Geometry: see drawing. Coordinates: mm, zero at the bounding-box minimum. A direction names the side the tool comes from. Coordinates: 2 decimals unless noted, no trailing zeros. Write each loop counter-clockwise with the first axis right and the second up, starting at its lowest first coordinate (ties: lowest second). Pieces come first, ordered by that corner, then holes. Notation, with made-up numbers: (7, 41) - (41, 41) arc R20 cw to (41, 76) - close; hole circle Ø8 at (86.25, 64.5). An arc over 180 degrees is marked (long way). One line per question, with ' | ' between items. Start each with the question number.
1) Line query: line 1 (Z direction, x = 22, y = 89.5); line 2 (Y direction, x = 24, z = 9); line 3 (Z direction, x = 4.5, y = 69.5). Output: solid intervals per line, ascending.
2) Section query D-D on x = 32.5. Return loops of the section in (y, z).
3) Section query C-C on z = 22.25. Return loops of the section in (x, y).
4) Section query A-A on y = 153. Return loops of the section in (x, z).
5) Reachability of the marked faces 1, 2 and 3 from +Z, -Z, +X, -X, +Y, -Y: full face, straight path, thin tool, end or side. Return the list, or none.
6) Section query B-B on x = 18.5. Return loops of the section in (y, z), and give its area (3 significant figures).
7) First-contact query: P1, Ø0.9, axis at x = 5, z = 16.5, coming from the +Y side; P2, Ø5, axis at x = 32.5, y = 139.5, coming from the +Z side; P3, Ø3, axis at x = 21, y = 161.5, coming from the +Z side. Flat tips, straight axial feed; report the tip coordinate or a pass-through.
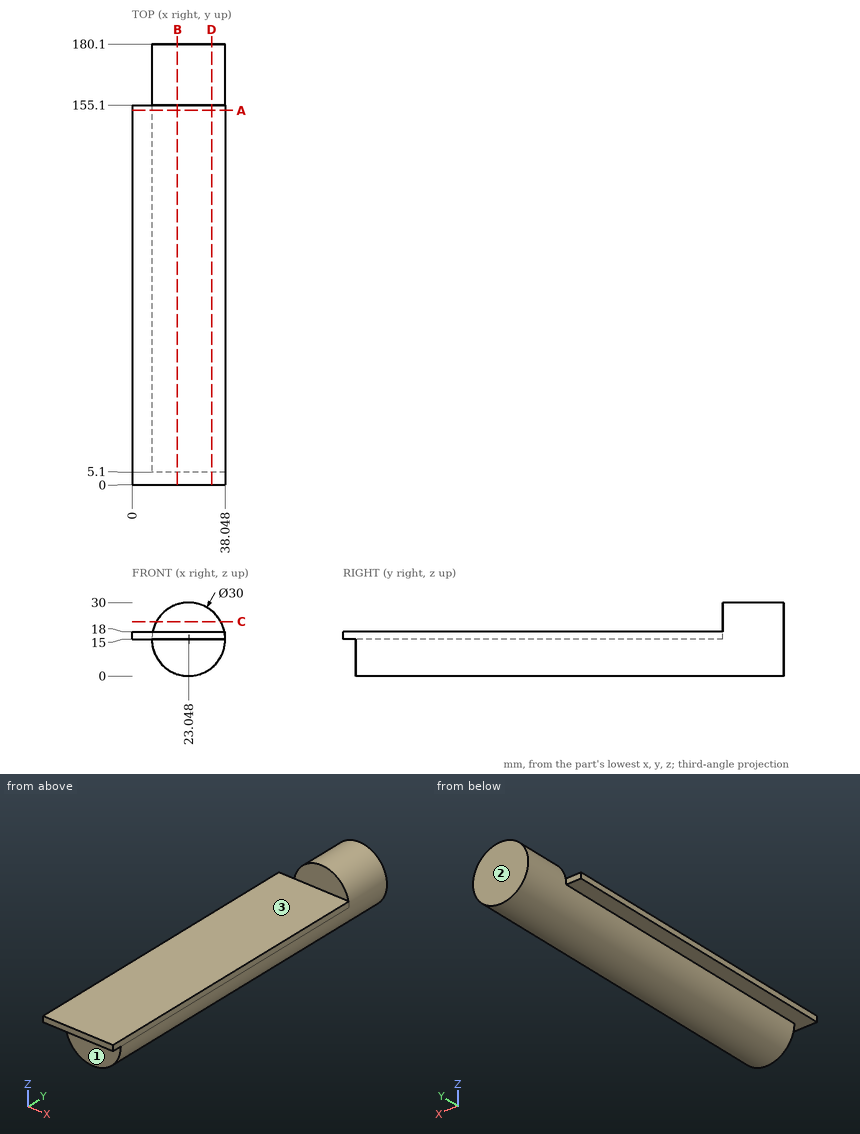
Answer key:
1) line 1: 0.04 to 18 | line 2: 5.1 to 180.1 | line 3: 15 to 18
2) outline: (0, 15) - (5.1, 15) - (5.1, 3.35) - (180.1, 3.35) - (180.1, 26.65) - (155.1, 26.65) - (155.1, 18) - (0, 18) - close
3) outline: (9.92, 155.1) - (36.18, 155.1) - (36.18, 180.1) - (9.92, 180.1) - close
4) outline: (0, 15) - (8.05, 15) arc R15 ccw to (38.05, 15) - (38.05, 18) - (0, 18) - close
5) face 1: -Z, +X, -X, -Y | face 2: +Z, -Z, +X, -X, +Y | face 3: +Z, +X, -X, -Y
6) outline: (0, 15) - (5.1, 15) - (5.1, 0.71) - (180.1, 0.71) - (180.1, 29.29) - (155.1, 29.29) - (155.1, 18) - (0, 18) - close | area: 3,320 mm²
7) P1: y = 155.1 | P2: z = 18 | P3: z = 29.99
